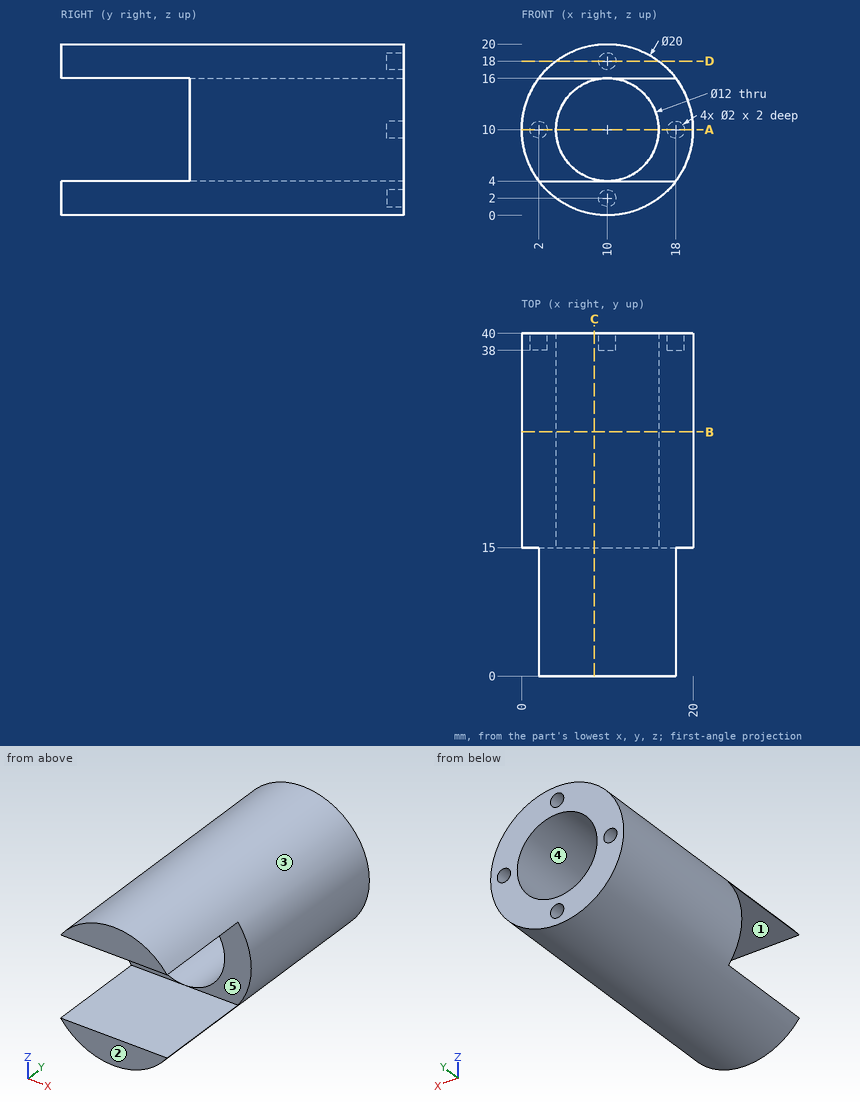
The figure shows three views and two pictorial views of one solid part (mm, origin at its lowest corner). Answer the questions. A direction names the side the tool comes from. Give positions to 0.01 mm unless a question says otherwise; leave off trailing zeros. Loops run counter-clockwise (first coordinate to the right, second up) from the corner with the lowest first, then second, coordinate; pieces in that order, holes last. Notation, with made-up numbers: (-11.75, 17.25) -> (42.25, 17.25) arc R28 cw to (42.25, 49.25) -> close; hole circle Ø5 at (76, 51). An arc over 180 degrees is marked (long way). Use a Markdown table: item, result. Add a question column.
1. Determine the mould class of the marked faces 3, 4 and 5 for opening direction X: released by +X, released by -X, zero draft, split by the parting line, or undercut.
2. Section D-D on z = 18 is taken. Determine the outline of the cut face in (x, y), and give its area (3 significant figures).
3. Section B-B on y = 28.5 is taken. Determine the outline of the cut face in (x, z), and give its area (3 significant figures).
4. Section C-C on x = 8.5 is taken. Determine the outline of the cut face in (y, z).
5. For the marked faces 1 and 2, determine the directions among +Z, -Z, +X, -X, +Y, -Y from which every point of the face is accessible in a straight line to the end or side of a thin tool.
6. Section A-A on z = 10 is taken. Determine the outline of the cut face in (x, y).
7. Flat-ended cylindrical pins translate along their axes: pin 1 Ø4 at (x, z) = (5, 7) entering from -Y; pin 2 Ø2.5 at (x, z) = (10, 2) entering from +Y; pin 3 Ø2 at (x, y) = (11.5, 19) entering from -Z; pin 4 Ø1.2 at (x, z) = (10, 18) entering from +Y. Find the tip coordinate at first contact, or state that the pin passes through.
8. Find the intervals of material crossed by probe 1 along X at (y, z) = (38.85, 10); probe 2 along X at (y, z) = (39.05, 18); probe 3 along X at (y, z) = (24.5, 9.75), in increasing order.
Results below:
| question | item | result |
|---|---|---|
| 1 | face 3 | split by the parting line |
| 1 | face 4 | undercut |
| 1 | face 5 | zero draft |
| 2 | outline | (4, 0) -> (16, 0) -> (16, 40) -> (11, 40) -> (11, 38) -> (9, 38) -> (9, 40) -> (4, 40) -> close |
| 2 | area | 476 mm^2 |
| 3 | outline | circle Ø20 at (10, 10); hole circle Ø12 at (10, 10) |
| 3 | area | 201 mm^2 |
| 4 | outline | (0, 0.11) -> (40, 0.11) -> (40, 4.19) -> (15, 4.19) -> (15, 4) -> (0, 4) -> close; (0, 16) -> (15, 16) -> (15, 15.81) -> (40, 15.81) -> (40, 19.89) -> (0, 19.89) -> close |
| 5 | face 1 | +X, -X, -Y |
| 5 | face 2 | +Z, -Z, +X, -X, -Y |
| 6 | outline | (0, 15) -> (4, 15) -> (4, 40) -> (3, 40) -> (3, 38) -> (1, 38) -> (1, 40) -> (0, 40) -> close; (16, 15) -> (20, 15) -> (20, 40) -> (19, 40) -> (19, 38) -> (17, 38) -> (17, 40) -> (16, 40) -> close |
| 7 | pin 1 | stops at y = 15 |
| 7 | pin 2 | stops at y = 40 |
| 7 | pin 3 | stops at z = 0.01 |
| 7 | pin 4 | stops at y = 38 |
| 8 | probe 1 | x = 0 to 1, 3 to 4, 16 to 17, 19 to 20 |
| 8 | probe 2 | x = 4 to 9, 11 to 16 |
| 8 | probe 3 | x = 0 to 4.01, 15.99 to 20 |
